Drawing for the job (mm, zero at the part's lowest x, y, z). Coordinates: 2 decimals unless noted, no trailing zeros. Order: outer loops, then holes, each group sorted by start corner. A loop starts at its lowest first (then second) coordinate and runs counter-clockwise, first axis right, second up. Notation, with made-up numbers: (53.25, 57.5) - (75.25, 57.5) arc R9 cw to (75.25, 66.5) - close; hole circle Ø3 at (-34, 28.5). An arc over 180 degrees is marked (long way). Put each result on its own line as item: value. Start each with the question number.
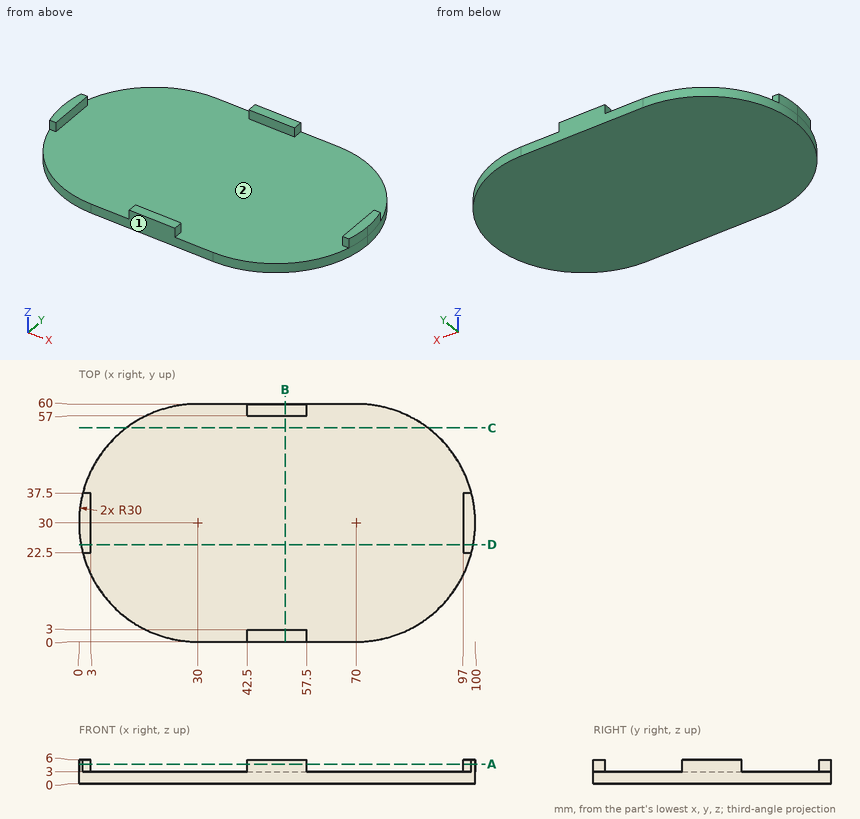
Item 1: Slice it at D-D, the plane y = 24.5. Give the cut face in (x, z), plus the area to 3 significant figures.
Item 2: Wall check: line 1 along X through (y, z) = (25.5, 4.8); line 2 along Z through (x, y) = (43.5, 34); line 3 along X through (y, z) = (35, 4.45). Give the ranges that are in metal, low to high.
Item 3: Slice it at C-C, the plane y = 54. Give the cut face in (x, z), plus the area to 3 significant figures.
Item 4: Slice it at B-B, the plane x = 52. Give the cut face in (y, z).
Item 5: Pull direction X, two halves, no side cores. Call the marked faces 1 and 2: pulls with the +X half, pulls with the -X half, needs draft (parallel to the pull), parting line crosses it, or undercut.
Item 6: Flat gauge pins, fed straight in: pin 1 Ø0.9 at (y, z) = (59, 4) entering from +X; pin 2 Ø0.6 at (x, z) = (2, 4.5) entering from -Y; pin 3 Ø2.5 at (x, z) = (1.5, 4.5) entering from +Y. Where does each tip first touch, or does it go through?
Item 7: Slice it at A-A, the plane z = 4.9. Give the cut face in (x, y), plus the area to 3 significant figures.
Here are the results:
1. outline: (0.51, 0) - (99.49, 0) - (99.49, 6) - (97, 6) - (97, 3) - (3, 3) - (3, 6) - (0.51, 6) - close
1. area: 312 mm^2
2. line 1: x = 0.34 to 3, 97 to 99.66
2. line 2: z = 0 to 3
2. line 3: x = 0.42 to 3, 97 to 99.58
3. outline: (12, 0) - (88, 0) - (88, 3) - (12, 3) - close
3. area: 228 mm^2
4. outline: (0, 0) - (60, 0) - (60, 6) - (57, 6) - (57, 3) - (3, 3) - (3, 6) - (0, 6) - close
5. face 1: needs draft
5. face 2: undercut
6. pin 1: stops at x = 57.5
6. pin 2: stops at y = 22.5
6. pin 3: stops at y = 37.5
7. outline: (0, 30) arc R30 ccw to (0.95, 22.5) - (3, 22.5) - (3, 37.5) - (0.95, 37.5) arc R30 ccw to start; (42.5, 0) - (57.5, 0) - (57.5, 3) - (42.5, 3) - close; (42.5, 57) - (57.5, 57) - (57.5, 60) - (42.5, 60) - close; (97, 22.5) - (99.05, 22.5) arc R30 ccw to (100, 30) arc R30 ccw to (99.05, 37.5) - (97, 37.5) - close
7. area: 171 mm^2
